```python
from build123d import *

# Parameters (mm, degrees)
F0_R     = 100
F0_R_2   = 99.5
F1_DEPTH = 50
F3_R     = 100
F3_R_2   = 99.5
F4_DEPTH = 200
F7_DEPTH = 222


with BuildPart() as f1:
    # F0 (on Front) → F1 (new body)
    with BuildSketch(Plane.XZ):
        Circle(F0_R)
        Circle(F0_R_2, mode=Mode.SUBTRACT)
    extrude(amount=F1_DEPTH)

    # F3 (on offset) → F4 (join)
    with BuildSketch(Plane.XZ.offset(50)):
        Circle(F3_R)
        Circle(F3_R_2, mode=Mode.SUBTRACT)
    extrude(amount=F4_DEPTH)

    # F6 (on offset) → F7 (cut)
    with BuildSketch(Plane.YZ.offset(100)):
        with BuildLine():
            add(Edge.make_bspline(
                [(-11.5396156907, 109.1770529747), (-37.40660144, 82.3029038002), (-74.6953320253, -14.6375859027), (-206.542273136, -48.3033385091), (-249.0700861085, -58.1255167434)],
                knots=[0, 0, 0, 0, 0.4686228188, 0.9205231007, 0.9205231007, 0.9205231007, 0.9205231007], degree=3))
            Line((-11.5396156907, 109.1770529747), (-268.6304729415, 109.1770529747))
            Line((-268.6304729415, 109.1770529747), (-269.2039608955, -62.7321824431))
            add(Edge.make_bspline(
                [(-249.0700861085, -58.1255167434), (-256.5495652028, -59.8529692417), (-263.3424316326, -61.3730310201), (-269.2039608955, -62.7321824431)],
                knots=[0.9205231007, 0.9205231007, 0.9205231007, 0.9205231007, 1, 1, 1, 1], degree=3))
        make_face()
        with BuildLine():
            ThreePointArc((-250.1155138016, -59.2780299485), (-249.7733014387, -58.5380431181), (-249.0700861085, -58.1255167434))
            add(Edge.make_bspline(
                [(-249.0700861085, -58.1255167434), (-256.5495652028, -59.8529692417), (-263.3424316326, -61.3730310201), (-269.2039608955, -62.7321824431)],
                knots=[0.9205231007, 0.9205231007, 0.9205231007, 0.9205231007, 1, 1, 1, 1], degree=3))
            Line((-269.2039608955, -62.7321824431), (-254.4201612473, -60.6556199491))
            Line((-254.4201612473, -60.6556199491), (-250.1155138016, -59.2780299485))
        make_face()
    extrude(amount=-F7_DEPTH, mode=Mode.SUBTRACT)


solid = f1.part
```
Geometry: final body of the model. Coordinates: model frame, mm. Coordinates: 2 decimals unless noted, no trailing zeros. Order: outer loops, then holes, each group sorted by start corner. A loop starts at its lowest first (then second) coordinate and runs counter-clockwise, first axis right, second up. Notation, with made-up numbers: (18.25, 60) -> (73.25, 60) arc R29 cw to (73.25, 86) -> close; hole circle Ø11 at (-38, -10.5). An arc over 180 degrees is marked (long way). Use CSV: the item, a comma, the result in double quotes.
1) Mould query, pull axis Z, two halves, no side actions, for faces 1 (the cylindrical face through (-21.57, -95.472, -97.134)), 2 (the cylindrical face through (-21.68, -95.47, -97.62)). Classes: +Z half, -Z half, draft (parallel to the pull), parting line (faces both ways), or undercut.
Findings:
face 1,"undercut"
face 2,"parting line"
2) Pin query (flat end, axial travel): pin 1 Ø10 at (x, y) = (-41.5, -210) entering from +Z; pin 2 Ø2 at (x, y) = (14.5, -189) entering from -Z; pin 3 Ø1.5 at (x, y) = (8, -88.5) entering from +Z. Return the tip coordinate at first contact, or that it passes through.
Findings:
pin 1,"stops at z = -87.97"
pin 2,"stops at z = -99.08"
pin 3,"stops at z = -99.11"
3) Section A-A on z = -78. Output: boundary loops of the cut face in (x, y).
Findings:
outline,"(-62.58, -250) -> (-61.78, -250) -> (-61.78, 0) -> (-62.58, 0) -> close; (61.78, -250) -> (62.58, -250) -> (62.58, 0) -> (61.78, 0) -> close"
4) Line query: line 1 (X direction, y = -96.5, z = -17); line 2 (X direction, y = -67.5, z = -75); line 3 (Z direction, x = 0, y = -71). Output: solid intervals per line, ascending.
Findings:
line 1,"x = -98.54 to -98.04, 98.04 to 98.54"
line 2,"x = -66.14 to -65.39, 65.39 to 66.14"
line 3,"z = -100 to -99.5"
